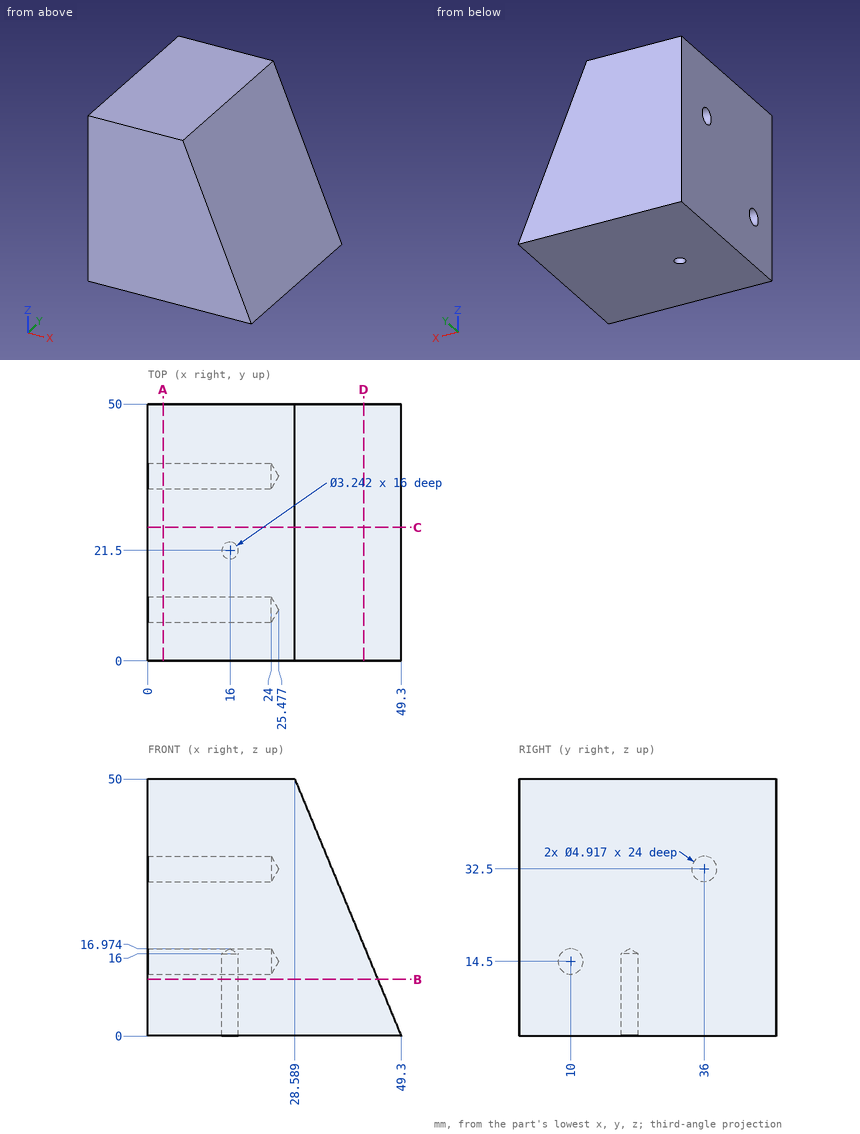
Source: three-view drawing plus pictorial views. Frame: mm from the lowest corner of the part. Give positions to 0.01 mm unless a question says otherwise; leave off trailing zeros. Write each loop counter-clockwise with the first axis right and the second up, starting at its lowest first coordinate (ties: lowest second). Pieces come first, ordered by that corner, then holes.
(1) Cut plane B-B, the plane z = 11. Return loops of the section in (x, y).
(2) Cut plane C-C, the plane y = 26. Return loops of the section in (x, z).
(3) Cut plane A-A, the plane x = 3. Return loops of the section in (y, z).
(4) Cut plane D-D, the plane x = 42. Return loops of the section in (y, z).
(5) Ray query, line 1 (Z direction, x = 14.5, y = 10); line 2 (Y direction, x = 8.25, z = 14.5); line 3 (Y direction, x = 16, z = 7). Return the intervals inside material, ascending.
(6) First-contact query: P1, Ø4.5, axis at y = 10, z = 14.5, coming from the +X side; P2, Ø6, axis at y = 44, z = 42, coming from the +X side (1 decimal); P3, Ø4, axis at x = 22, z = 24.5, coming from the -Y side; P4, Ø8, axis at y = 22.5, z = 29, coming from the +X side (1 decimal). Flat tips, straight axial feed; report the tip coordinate or a pass-through.
Values follow:
1. outline: (0, 0) - (44.74, 0) - (44.74, 50) - (0, 50) - close; hole circle Ø3.24 at (16, 21.5)
2. outline: (0, 0) - (49.3, 0) - (28.59, 50) - (0, 50) - close
3. outline: (0, 0) - (50, 0) - (50, 50) - (0, 50) - close; hole circle Ø4.92 at (10, 14.5); hole circle Ø4.92 at (36, 32.5)
4. outline: (0, 0) - (50, 0) - (50, 17.62) - (0, 17.62) - close
5. line 1: z = 0 to 12.04, 16.96 to 50
5. line 2: y = 0 to 7.54, 12.46 to 50
5. line 3: y = 0 to 19.88, 23.12 to 50
6. P1: stops at x = 44.23
6. P2: stops at x = 33.1
6. P3: stops at y = 0
6. P4: stops at x = 38.9
